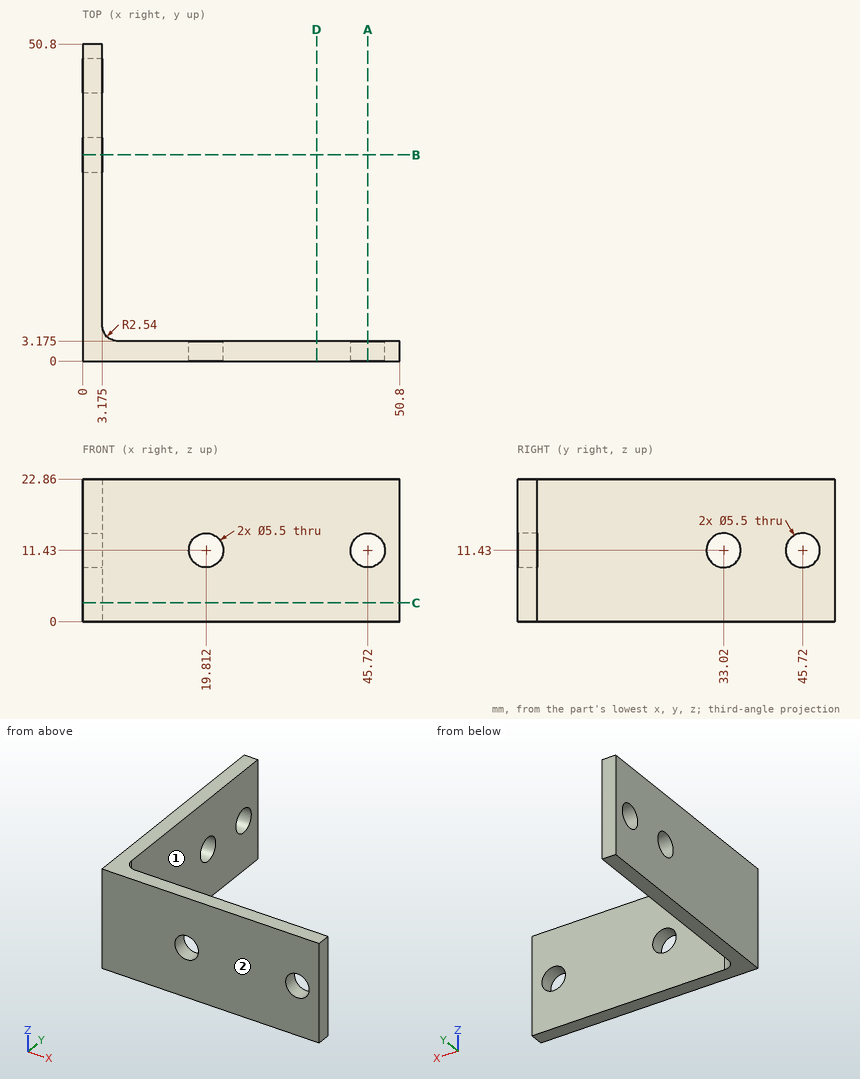
For this review, use the dimensioned drawing (mm, ordinates from the lowest corner) and the shaded views. A direction names the side the tool comes from. Round coordinates to 2 decimals unless told otherwise and drop trailing zeros. Loops run counter-clockwise (first coordinate to the right, second up) from the corner with the lowest first, then second, coordinate; pieces in that order, holes last. Notation, with made-up numbers: (89, 85.25) -> (109, 85.25) arc R10 cw to (109, 97.25) -> close; hole circle Ø5 at (-2, 65.5). An arc over 180 degrees is marked (long way). Write item = value, one per line. Start each with the question number.
Item 1: To check wall thickness, follow L1, parallel to X at y = 1.35, z = 11.43; L2, parallel to Z at x = 1.5, y = 45.72; L3, parallel to Y at x = 48, z = 13.25 (3 decimals). State the ranges of each line that lie inside material, in increasing order.
Item 2: For the marked faces 1 and 2, list the 3-axis set-ups (+Z, -Z, +X, -X, +Y, -Y) from which the entire face can be reached by the end or side of a thin tool; tool diameter is ignored.
Item 3: Take a section at A-A on x = 45.72. Give the boundary of the cut face in (y, z) (3 decimals), plus the area to 3 significant figures.
Item 4: Insertion check: pin 1 (5 mm diameter, centred on x = 6, y = 7, fed in from +Z); pin 2 (7 mm diameter, centred on x = 36.5, z = 6, fed in from +Y) (3 decimals); pin 3 (7 mm diameter, centred on y = 33.02, z = 11.43, fed in from +X) (3 decimals). Each pin has a flat end and moves straight along its axis. Give the tip position at first contact, or say it passes through.
Item 5: Take a section at D-D on x = 37.5. Give the boundary of the cut face in (y, z) (3 decimals).
Item 6: Take a section at C-C on z = 3. Give the boundary of the cut face in (x, y) (3 decimals), plus the area to 3 significant figures.
Result:
q1.L1 = 0 to 17.06, 22.56 to 42.97, 48.47 to 50.8
q1.L2 = 0 to 8.68, 14.18 to 22.86
q1.L3 = 0 to 3.175
q2.face_1 = +Z, -Z, +X, +Y
q2.face_2 = +Z, -Z, +X, -X, -Y
q3.outline = (0, 0) -> (3.175, 0) -> (3.175, 8.68) -> (0, 8.68) -> close; (0, 14.18) -> (3.175, 14.18) -> (3.175, 22.86) -> (0, 22.86) -> close
q3.area = 55.1 mm²
q4.pin_1 = through
q4.pin_2 = 3.175
q4.pin_3 = 3.175
q5.outline = (0, 0) -> (3.175, 0) -> (3.175, 22.86) -> (0, 22.86) -> close
q6.outline = (0, 0) -> (50.8, 0) -> (50.8, 3.175) -> (5.715, 3.175) arc R2.54 cw to (3.175, 5.715) -> (3.175, 50.8) -> (0, 50.8) -> close
q6.area = 314 mm²
